from build123d import *

# Parameters (mm, degrees)
SKETCH1_R           = 1.449961854
SKETCH1_R_2         = 1.45
SKETCH1_W           = 3.400011
SKETCH1_H           = 6.199989
BOSS_EXTRUDE2_DEPTH = 5.85


with BuildPart() as part:
    # Sketch1 → Boss-Extrude2 (new body)
    with BuildSketch(Plane.XY):
        with BuildLine():
            Line((389.265872387, 564.138903138), (411.155971541, 564.138903138))
            ThreePointArc((411.155971541, 564.138903138), (412.46753945, 563.584161878), (412.982994127, 562.256662455))
            ThreePointArc((412.982994127, 562.256662455), (416.531053859, 553.119006976), (425.559046996, 549.30052358))
            ThreePointArc((425.559046996, 549.30052358), (428.720667438, 546.138903138), (425.559046996, 542.977282695))
            ThreePointArc((425.559046996, 542.977282695), (416.910383014, 539.55653755), (412.941547102, 531.145281549))
            ThreePointArc((412.941547102, 531.145281549), (412.268542883, 529.718966402), (410.801969943, 529.138903138))
            Line((410.801969943, 529.138903138), (389.265871713, 529.138903138))
            add(Edge.make_bspline(
                [(387.560996, 530.842035377), (387.467163743, 529.138903138), (389.265871713, 529.138903138)],
                knots=[0, 0, 0, 1, 1, 1], degree=2))
            Line((387.560996, 530.842035377), (387.560996, 562.435769381))
            add(Edge.make_bspline(
                [(387.560996, 562.435769381), (387.467162762, 564.138903138), (389.265872387, 564.138903138)],
                knots=[0, 0, 0, 1, 1, 1], degree=2))
        make_face()
        with Locations((425.559046996, 546.138903138)):
            Circle(SKETCH1_R, mode=Mode.SUBTRACT)
        with Locations((399.559046996, 534.238897638)):
            Circle(SKETCH1_R_2, mode=Mode.SUBTRACT)
        Polygon((405.698755359, 552.338914138), (405.698755359, 554.938914138), (408.557097991, 554.938914138), (408.557097991, 561.138903138), (402.757097991, 561.138903138), (402.757097991, 554.938914138), (396.360996, 554.938914138), (396.360996, 561.138903138), (390.560996, 561.138903138), (390.560996, 554.938914138), (393.683007359, 554.938914138), (393.683007359, 552.338914138), align=None, mode=Mode.SUBTRACT)
        with Locations((394.409041496, 534.238897638)):
            Rectangle(SKETCH1_W, SKETCH1_H, mode=Mode.SUBTRACT)
        with Locations((404.709052496, 534.238897638)):
            Rectangle(SKETCH1_W, SKETCH1_H, mode=Mode.SUBTRACT)
        with BuildLine():
            Line((396.188262357, 549.638903138), (413.915690223, 549.638903138))
            ThreePointArc((413.915690223, 549.638903138), (417.415690223, 546.138903138), (413.915690223, 542.638903138))
            Line((413.915690223, 542.638903138), (396.188262357, 542.638903138))
            ThreePointArc((396.188262357, 542.638903138), (392.688262357, 546.138903138), (396.188262357, 549.638903138))
        make_face(mode=Mode.SUBTRACT)
    extrude(amount=BOSS_EXTRUDE2_DEPTH)


solid = part.part
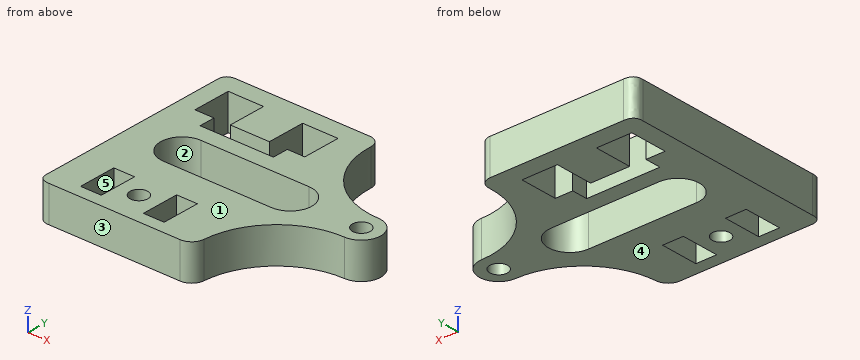
Source: CAD feature listing. Evaluate the final solid. Frame: model axes, mm. Face numbers are marked on the shaded views. A direction names the side the tool comes from. Round coordinates to 2 decimals unless told otherwise and drop trailing zeros. Order: outer loops, then holes, each group sorted by start corner. A loop starts at its lowest first (then second) coordinate and runs counter-clockwise, first axis right, second up. Notation, with made-up numbers: (87.5, -38.5) - (134.5, -38.5) arc R14 cw to (134.5, -30.5) - close; hole circle Ø1 at (-10.5, 39). An arc over 180 degrees is marked (long way). Use a Markdown table: item, result. Add a question column.
1. Set-up query: the marked faces 1 and 2. Return all of +Z, -Z, +X, -X, +Y, -Y with unobstructed straight access to the full face (end or side cutting, diameter ignored); none if empty.
2. Line query: probe 1 along Y at (x, z) = (401.5, 5.2); probe 2 along X at (y, z) = (560, 2.2); probe 3 along X at (y, z) = (546.5, 1.7). Output: solid intervals per line, ascending.
3. Mould query, pull axis Y, two halves, no side actions, for the marked faces 3, 4 and 5. Classes: +Y half, -Y half, draft (parallel to the pull), parting line (faces both ways), or undercut.
4. First-contact query: pin 1 (2 mm diameter, centred on x = 416, z = 5, fed in from +Y); pin 2 (1.8 mm diameter, centred on y = 535, z = 2, fed in from +X); pin 3 (3 mm diameter, centred on y = 535.5, z = 2.5, fed in from +X). Flat tips, straight axial feed; report the tip coordinate or a pass-through.
5. Section query D-D (x = 426). Return the cut outline in (y, z).
6. Section query B-B (y = 560). Return the cut outline in (x, z).
7. Section query C-C (x = 395.5). Return the cut outline in (y, z), then the cut area to 3 significant figures.
8. Section query A-A (x = 402). Return the cut outline in (y, z).
Derived:
| question | item | result |
|---|---|---|
| 1 | face 1 | +Z, +X, -X, +Y, -Y |
| 1 | face 2 | +Z, -Z |
| 2 | probe 1 | 529.14 to 542.64, 549.64 to 552.34, 554.94 to 564.14 |
| 2 | probe 2 | 387.56 to 390.56, 396.36 to 402.76, 408.56 to 413.12 |
| 2 | probe 3 | 387.56 to 392.71, 417.4 to 424.15, 426.96 to 428.7 |
| 3 | face 3 | -Y half |
| 3 | face 4 | draft |
| 3 | face 5 | undercut |
| 4 | pin 1 | y = 555.04 |
| 4 | pin 2 | x = 414.21 |
| 4 | pin 3 | x = 414.82 |
| 5 | outline | (543.01, 0) - (544.76, 0) - (544.76, 5.85) - (543.01, 5.85) - close; (547.52, 0) - (549.27, 0) - (549.27, 5.85) - (547.52, 5.85) - close |
| 6 | outline | (387.56, 0) - (390.56, 0) - (390.56, 5.85) - (387.56, 5.85) - close; (396.36, 0) - (402.76, 0) - (402.76, 5.85) - (396.36, 5.85) - close; (408.56, 0) - (413.12, 0) - (413.12, 5.85) - (408.56, 5.85) - close |
| 7 | outline | (529.14, 0) - (531.14, 0) - (531.14, 5.85) - (529.14, 5.85) - close; (537.34, 0) - (542.71, 0) - (542.71, 5.85) - (537.34, 5.85) - close; (549.57, 0) - (552.34, 0) - (552.34, 5.85) - (549.57, 5.85) - close; (561.14, 0) - (564.14, 0) - (564.14, 5.85) - (561.14, 5.85) - close |
| 7 | area | 76.8 mm2 |
| 8 | outline | (529.14, 0) - (542.64, 0) - (542.64, 5.85) - (529.14, 5.85) - close; (549.64, 0) - (552.34, 0) - (552.34, 5.85) - (549.64, 5.85) - close; (554.94, 0) - (564.14, 0) - (564.14, 5.85) - (554.94, 5.85) - close |
